The model under review builds one solid part; all positions refer to its coordinate system, in mm. Face numbers are marked on the shaded views. A direction names the side the tool comes from. Round coordinates to 2 decimals unless told otherwise and drop trailing zeros. Write each loop counter-clockwise with the first axis right and the second up, starting at its lowest first coordinate (ties: lowest second). Pieces come first, ordered by that corner, then holes.
Item 1: Add section A-A (x = -158). Give the boundary of the cut face in (y, z).
Item 2: Clearance check with flat-ended pins moving along their axes: pin 1 Ø15 at (y, z) = (-8.5, -227) entering from -X; pin 2 Ø8 at (x, y) = (-359.5, -32) entering from +Z; pin 3 Ø11.5 at (x, y) = (-756, 4.5) entering from +Z. State where each tip first meets the part, or that it passes through.
Item 3: Machinability: for the marked faces 1 and 2, which of the approach directions +Z, -Z, +X, -X, +Y, -Y give a long, thin tool a straight path to every point of the face, cutting with its end or side? Answer none if there is none.
Item 4: Add section C-C (z = -249). Give the boundary of the cut face in (x, y).
Item 5: Add section B-B (z = -169). Give the boundary of the cut face in (x, y), plus the area to 3 significant figures.
Item 6: To check wall thickness, follow L1, parallel to Z at x = 493, y = 26; L2, parallel to Y at x = 264, z = -33; L3, parallel to X at y = 11.5, z = -240.5. State the ranges of each line that lie inside material, in increasing order.
```python
from build123d import *

# Parameters (mm, degrees)
F1_DEPTH = 19
F3_DEPTH = 811


with BuildPart() as f1:
    # F0 (on Front) → F1 (new body, symmetric)
    with BuildSketch(Plane.XZ):
        Polygon((711, 0), (0, 0), (-711, 0), (-711, -19), (-811, -19), (-811, -213), (-775, -213), (-775, -232), (-793, -232), (-793, -282), (0, -282), (793, -282), (793, -232), (775, -232), (775, -213), (811, -213), (811, -19), (711, -19), align=None)
    extrude(amount=F1_DEPTH, both=True)

    # F2 (on Right) → F3 (join, symmetric)
    with BuildSketch(Plane.YZ):
        Polygon((38, -42), (-38, -42), (-38, -61), (-28, -61), (-28, -89), (-38, -89), (-38, -108), (38, -108), (38, -89), (28, -89), (28, -61), (38, -61), align=None)
    extrude(amount=F3_DEPTH, both=True)


solid = f1.part
```
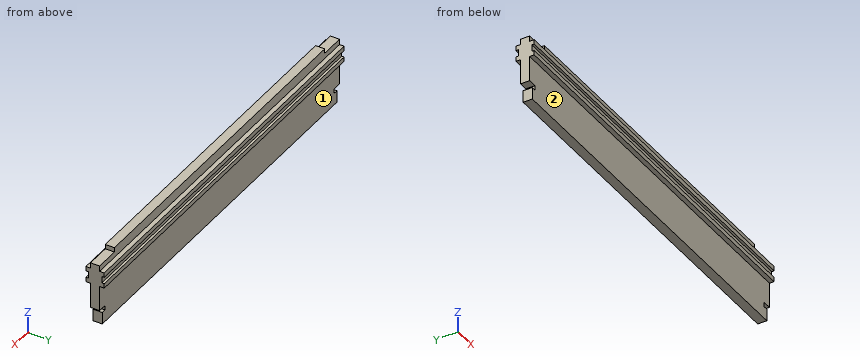
Numbers:
1. outline: (-38, -108) - (-19, -108) - (-19, -282) - (19, -282) - (19, -108) - (38, -108) - (38, -89) - (28, -89) - (28, -61) - (38, -61) - (38, -42) - (19, -42) - (19, 0) - (-19, 0) - (-19, -42) - (-38, -42) - (-38, -61) - (-28, -61) - (-28, -89) - (-38, -89) - close
2. pin 1: stops at x = -793
2. pin 2: stops at z = -42
2. pin 3: stops at z = -19
3. face 1: -Z, +X, -X, +Y
3. face 2: -Z, +X, -X, -Y
4. outline: (-793, -19) - (793, -19) - (793, 19) - (-793, 19) - close
5. outline: (-811, -19) - (811, -19) - (811, 19) - (-811, 19) - close
5. area: 61,600 mm2
6. L1: z = -108 to -42
6. L2: y = -19 to 19
6. L3: x = -793 to 793
